from build123d import *

# Parameters (mm, degrees)
F0_R     = 47.5
F1_DEPTH = 1
F2_R     = 47.5
F2_R_2   = 46.5
F3_DEPTH = 4
F4_R     = 21.25
F4_R_2   = 20.25
F5_DEPTH = 5
F6_R     = 3.5
F6_R_2   = 5
F7_DEPTH = 25
F8_R     = 1.5
F9_DEPTH = 25


with BuildPart() as f1:
    # F0 (on Top) → F1 (new body)
    with BuildSketch(Plane.XY):
        Circle(F0_R)
    extrude(amount=F1_DEPTH)

    # F2 (on face) → F3 (join)
    with BuildSketch(Plane.XY.offset(1)):
        Circle(F2_R)
        Circle(F2_R_2, mode=Mode.SUBTRACT)
    extrude(amount=F3_DEPTH)

    # F4 (on face) → F5 (join)
    with BuildSketch(Plane.XY.offset(1)):
        Circle(F4_R)
        Circle(F4_R_2, mode=Mode.SUBTRACT)
    extrude(amount=F5_DEPTH)

    # F6 (on face) → F7 (cut)
    with BuildSketch(Plane.XY.offset(1)):
        with Locations((-7.818315, 6.234898)):
            Circle(F6_R)
        with Locations((-9.749279, -2.225209)):
            Circle(F6_R)
        with Locations((-4.338837, -9.009689)):
            Circle(F6_R)
        with Locations((4.338837, -9.009689)):
            Circle(F6_R)
        with Locations((9.749279, -2.225209)):
            Circle(F6_R)
        with Locations((7.818315, 6.234898)):
            Circle(F6_R)
        with Locations((0, 10)):
            Circle(F6_R)
        Circle(F6_R_2)
    extrude(amount=-F7_DEPTH, mode=Mode.SUBTRACT)

    # F8 (on face) → F9 (cut)
    with BuildSketch(Plane.XY.offset(1)):
        with Locations((-34, 0)):
            Circle(F8_R)
        with Locations((34, 0)):
            Circle(F8_R)
    extrude(amount=-F9_DEPTH, mode=Mode.SUBTRACT)


with BuildPart() as f10_1:
    # F10: copy of F1
    add(f1.part)


solid = f1.part
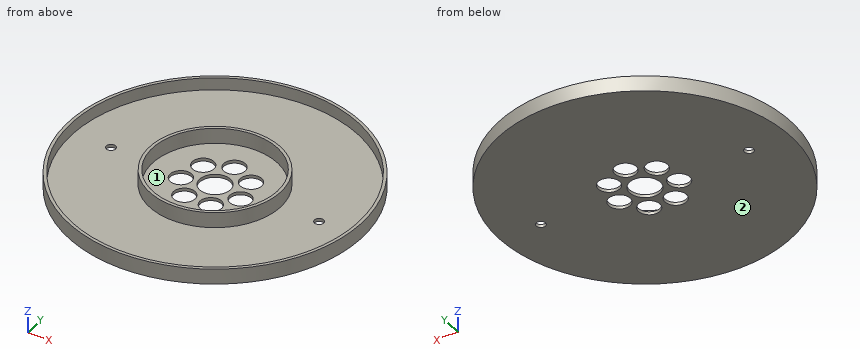
The listing builds one solid part. Answer for the finished solid, in the listing's coordinates (mm). Face numbers are marked on the shaded views. Give positions to 0.01 mm unless a question says otherwise; leave off trailing zeros. Write each loop counter-clockwise with the first axis right and the second up, starting at its lowest first coordinate (ties: lowest second). Pieces come first, ordered by that corner, then holes. Notation, with made-up numbers: (-4.75, 3) - (20.25, 3) arc R23 ccw to (20.25, 15) - close; hole circle Ø5 at (-17, 71). An arc over 180 degrees is marked (long way). One line per question, with ' | ' between items. Start each with the question number.
1. Section C-C, the plane y = -30.5 is taken. Determine the outline of the cut face in (x, z).
2. Given P1, Ø6, axis at x = -7, y = 10, coming from the +Z side; P2, Ø10, axis at x = 5, y = 7, coming from the -Z side; P3, Ø2, axis at y = -24.5, z = 4.5, coming from the -X side, each flat-ended and moving along its own axis, determine where each tip first touches the part or whether it passes through.
3. Straight lines are drawn through the part: line 1 (Y direction, x = 0, z = 0.55); line 2 (Y direction, x = -5, z = 1.05); line 3 (Z direction, x = -43, y = 17). For each, find the intervals that lie inside material, in ascending order.
4. Section B-B, the plane x = -34 is taken. Determine the outline of the cut face in (y, z), then the cut area to 3 significant figures.
5. Section A-A, the plane z = 2.15 is taken. Determine the outline of the cut face in (x, y).
6. Determine the mould class of the marked faces 1 and 2 for opening direction Y: +Y half, -Y half, draft (parallel to the pull), parting line (faces both ways), or undercut.
7. Section D-D, the plane y = 0 is taken. Count the separate pieces of the cut face and the enclosed holes in it, then the cut area to 3 significant figures.
Result:
1) outline: (-36.41, 0) - (36.41, 0) - (36.41, 5) - (35.1, 5) - (35.1, 1) - (-35.1, 1) - (-35.1, 5) - (-36.41, 5) - close
2) P1: stops at z = 1 | P2: stops at z = 0 | P3: stops at x = -41.28
3) line 1: y = -47.5 to -5, 5 to 6.5, 13.5 to 47.5 | line 2: y = -47.24 to -46.23, -20.65 to -19.62, 19.62 to 20.65, 46.23 to 47.24 | line 3: z = 0 to 1
4) outline: (-33.17, 0) - (-1.5, 0) - (-1.5, 1) - (-31.72, 1) - (-31.72, 5) - (-33.17, 5) - close; (1.5, 0) - (33.17, 0) - (33.17, 5) - (31.72, 5) - (31.72, 1) - (1.5, 1) - close | area: 74.9 mm2
5) outline: circle Ø95 at (0, 0); circle Ø42.5 at (0, 0); hole circle Ø93 at (0, 0); hole circle Ø40.5 at (0, 0)
6) face 1: undercut | face 2: draft
7) separate pieces: 6 | enclosed holes: 0 | area: 86.2 mm2
